Build history of the part. All positions in model axes, mm. Face numbers are marked on the shaded views. Give positions to 0.01 mm unless a question says otherwise; leave off trailing zeros. Write each loop counter-clockwise with the first axis right and the second up, starting at its lowest first coordinate (ties: lowest second). Pieces come first, ordered by that corner, then holes. Notation, with made-up numbers: (64, 24.25) -> (112, 24.25) arc R8 cw to (112, 37.25) -> close; hole circle Ø9 at (13.5, 28). An arc over 180 degrees is marked (long way). Put each result on its own line as item: value. Start each with the question number.
Item 1: Drill centre lines: line 1 along X through (y, z) = (0, 56); line 2 along Y through (x, z) = (100, 28); line 3 along X through (y, z) = (13, 67). Where is each one in solid material? Low to high.
Item 2: Slice it at A-A, the plane y = 0. List the corners of the cut face in (x, z), plus the area to 3 significant figures.
Item 3: Flat gauge pins, fed straight in: pin 1 Ø4.5 at (x, y) = (100, 0) entering from +Z; pin 2 Ø4 at (y, z) = (-5.5, 23.5) entering from +X; pin 3 Ø10 at (y, z) = (-9, 33) entering from -X; pin 4 Ø1 at (y, z) = (8, 54) entering from -X. Where does each tip first touch, or does it go through?
Item 4: Two-plate mould, pull along Y, no slides. Class the marked faces 1, 2, 3 and 4: pulls with the +Y half, pulls with the -Y half, needs draft (parallel to the pull), parting line crosses it, or undercut.
Item 5: Slice it at B-B, the plane z = 52. List the corners of the cut face in (x, y).
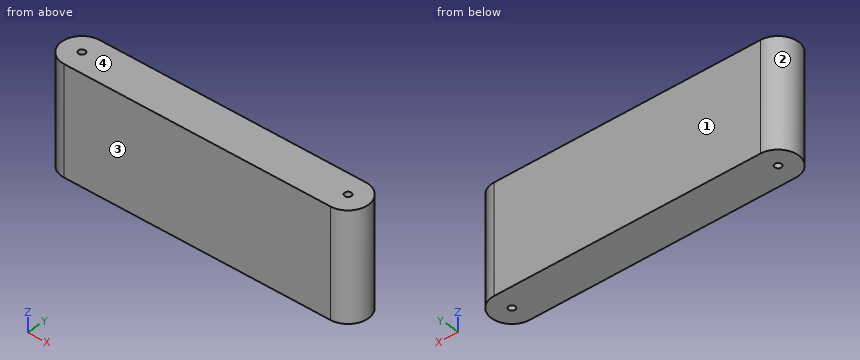
```python
from build123d import *

# Parameters (mm, degrees)
EXTRUDE_1_DEPTH          = 80
CUT_EXTRUDE_1_DEPTH      = 141.890028036
CUT_EXTRUDE_1_DEPTH_BACK = 141.890028036
SKETCH_2_R               = 2.5


with BuildPart() as part:
    # 草图1 → 凸台-拉伸1 (new body)
    with BuildSketch(Plane.XY):
        with BuildLine():
            Line((-100, 15), (100, 15))
            ThreePointArc((100, 15), (115, 0), (100, -15))
            Line((100, -15), (-100, -15))
            ThreePointArc((-100, -15), (-115, 0), (-100, 15))
        make_face()
    extrude(amount=EXTRUDE_1_DEPTH)

    # 草图2 → 切除-拉伸1 (cut, two sides: drawn at the far end of the back side and taken through both)
    with BuildSketch(Plane.XY.offset(80).offset(-CUT_EXTRUDE_1_DEPTH_BACK)):
        with Locations((-100, 0)):
            Circle(SKETCH_2_R)
        with Locations((100, 0)):
            Circle(SKETCH_2_R)
    extrude(amount=CUT_EXTRUDE_1_DEPTH + CUT_EXTRUDE_1_DEPTH_BACK, mode=Mode.SUBTRACT)


solid = part.part
```
Values follow:
1. line 1: -115 to -102.5, -97.5 to 97.5, 102.5 to 115
1. line 2: -15 to -2.5, 2.5 to 15
1. line 3: -107.48 to 107.48
2. outline: (-115, 0) -> (-102.5, 0) -> (-102.5, 80) -> (-115, 80) -> close; (-97.5, 0) -> (97.5, 0) -> (97.5, 80) -> (-97.5, 80) -> close; (102.5, 0) -> (115, 0) -> (115, 80) -> (102.5, 80) -> close
2. area: 17,600 mm2
3. pin 1: through
3. pin 2: x = 114.59
3. pin 3: x = -114.46
3. pin 4: x = -112.99
4. face 1: pulls with the +Y half
4. face 2: parting line crosses it
4. face 3: pulls with the -Y half
4. face 4: needs draft
5. outline: (-100, -15) -> (100, -15) arc R15 ccw to (100, 15) -> (-100, 15) arc R15 ccw to start; hole circle Ø5 at (-100, 0); hole circle Ø5 at (100, 0)
